from build123d import *

# Parameters (mm, degrees)
BOSS_EXTRUDE1_DEPTH = 10
BOSS_EXTRUDE2_DEPTH = 10
SKETCH3_W           = 10
SKETCH3_H           = 20
BOSS_EXTRUDE3_DEPTH = 20


with BuildPart() as part:
    # Sketch1 → Boss-Extrude1 (new body)
    with BuildSketch(Plane.XY):
        with BuildLine():
            Line((-75, 0), (75, 0))
            Line((75, 0), (75, -50.8))
            Line((75, -50.8), (71.214043559, -50.8))
            ThreePointArc((71.214043559, -50.8), (0, -10), (-71.214043559, -50.8))
            Line((-71.214043559, -50.8), (-75, -50.8))
            Line((-75, -50.8), (-75, 0))
        make_face()
    extrude(amount=BOSS_EXTRUDE1_DEPTH)

    # Sketch2 → Boss-Extrude2 (add)
    with BuildSketch(Plane.XY.offset(10)):
        with BuildLine():
            Line((75, 0), (75, -49.913046695))
            ThreePointArc((75, -49.913046695), (45.953391498, -19.534963213), (6, -6.486594379))
            ThreePointArc((6, -6.486594379), (4.927947794, -12.515421427), (5.368573056, -18.622949642))
            Line((5.368573056, -18.622949642), (3.627612554, -19.318821125))
            ThreePointArc((3.627612554, -19.318821125), (1.458266232, -12.897160035), (0, -6.277699769))
            ThreePointArc((0, -6.277699769), (-1.458266232, -12.897160035), (-3.627612554, -19.318821125))
            Line((-3.627612554, -19.318821125), (-5.368573056, -18.622949642))
            ThreePointArc((-5.368573056, -18.622949642), (-4.927947794, -12.515421427), (-6, -6.486594379))
            ThreePointArc((-6, -6.486594379), (-45.953391498, -19.534963213), (-75, -49.913046695))
            Line((-75, -49.913046695), (-75, 0))
            Line((-75, 0), (75, 0))
        make_face()
    extrude(amount=BOSS_EXTRUDE2_DEPTH)

    # Sketch3 → Boss-Extrude3 (add)
    with BuildSketch(Plane.XY.offset(20)):
        with Locations((-80, 0)):
            Rectangle(SKETCH3_W, SKETCH3_H)
    extrude(amount=-BOSS_EXTRUDE3_DEPTH)


solid = part.part
Geometry: final body of the model. Coordinates: model frame, mm. A direction names the side the tool comes from. Give positions to 0.01 mm unless a question says otherwise; leave off trailing zeros. Write each loop counter-clockwise with the first axis right and the second up, starting at its lowest first coordinate (ties: lowest second). Pieces come first, ordered by that corner, then holes. Notation, with made-up numbers: (-32.5, 30.5) -> (-27.5, 30.5) arc R17 cw to (-27.5, 43.5) -> close; hole circle Ø3 at (81, 84.25). An arc over 180 degrees is marked (long way). Answer as a JSON object with one key per item and string values.
1. Access query for faces 1 (the cylindrical face through (46.455, -19.853, 14.93)), 2 (the flat face through (75, -25, 10)), 3 (the cylindrical face through (-4.924, -12.601, 14.93)), 4 (the flat face through (-75, 5, 10)), 5 (the flat face through (-80, -10, 10)). Directions: +Z, -Z, +X, -X, +Y, -Y. A direction counts if a zero-diameter tool reaches every point of the face in a straight line with its end or side. Return the directions, or none.
Ans:
{"face 1": "+Z, -Y", "face 2": "+Z, -Z, +X, +Y, -Y", "face 3": "+Z", "face 4": "+Z, -Z, +X, +Y", "face 5": "+Z, -Z, -X, -Y"}
2. Contact query for flat-ended pins moving along their axis: pin 1 (1.5 mm diameter, centred on x = 3, y = -21, fed in from -Z); pin 2 (6 mm diameter, centred on y = -19, z = 12.5, fed in from -X); pin 3 (8 mm diameter, centred on x = 53, z = 2.5, fed in from +Y); pin 4 (4 mm diameter, centred on x = -46.5, y = -23.5, fed in from +Z). Output: stop coordinate, or through.
Ans:
{"pin 1": "passes through", "pin 2": "stops at x = -75", "pin 3": "stops at y = 0", "pin 4": "stops at z = 10"}
3. Cut plane C-C on x = 48.5. Output: boundary loops of the cut face in (y, z).
Ans:
{"outline": "(-25.75, 0) -> (0, 0) -> (0, 20) -> (-21.2, 20) -> (-21.2, 10) -> (-25.75, 10) -> close"}
4. Ray query, probe 1 along Z at (x, y) = (-57.5, -29); probe 2 along X at (y, z) = (-33, 4.75); probe 3 along X at (y, z) = (6, 7.75). Return the intervals inside material, ascending. Write a range as from..to.
Ans:
{"probe 1": "z = 0..10", "probe 2": "x = -75..-57.17, 57.17..75", "probe 3": "x = -85..-75"}
5. Cut plane A-A on y = -30.5. Output: boundary loops of the cut face in (x, z).
Ans:
{"outline": "(-75, 0) -> (-54.45, 0) -> (-54.45, 10) -> (-59.94, 10) -> (-59.94, 20) -> (-75, 20) -> close; (54.45, 0) -> (75, 0) -> (75, 20) -> (59.94, 20) -> (59.94, 10) -> (54.45, 10) -> close"}
6. Cut plane B-B on z = 3.5. Output: boundary loops of the cut face in (x, y).
Ans:
{"outline": "(-85, -10) -> (-75, -10) -> (-75, -50.8) -> (-71.21, -50.8) arc R82.55 cw to (71.21, -50.8) -> (75, -50.8) -> (75, 0) -> (-75, 0) -> (-75, 10) -> (-85, 10) -> close"}
7. Cut plane D-D on y = -43.5. Output: boundary loops of the cut face in (x, z).
Ans:
{"outline": "(-75, 0) -> (-66.4, 0) -> (-66.4, 10) -> (-70.97, 10) -> (-70.97, 20) -> (-75, 20) -> close; (66.4, 0) -> (75, 0) -> (75, 20) -> (70.97, 20) -> (70.97, 10) -> (66.4, 10) -> close"}
